Here's how the part is built. I have some questions about the finished solid (model axes, mm). A direction names the side the tool comes from. Round coordinates to 2 decimals unless told otherwise and drop trailing zeros. Write each loop counter-clockwise with the first axis right and the second up, starting at its lowest first coordinate (ties: lowest second). Pieces come first, ordered by that corner, then holes. Notation, with made-up numbers: (51.25, -36.75) -> (57.25, -36.75) arc R20 ccw to (57.25, -15.75) -> close; hole circle Ø10 at (82.5, -28.5). An arc over 180 degrees is marked (long way). Put each result on its own line as item: value. Start each with the question number.
1. I need wall thicknesses on probe 1 along X at (y, z) = (-22, 2.75); probe 2 along X at (y, z) = (-25, 3); probe 3 along X at (y, z) = (-21, 5.75). Which ranges of each line are inside material? Lowest first, please. Write a range as from..to.
2. For pin 1 (3 mm diameter, centred on x = -22.5, z = 5.5, fed in from -Y); pin 2 (1 mm diameter, centred on y = 20.5, z = 1, fed in from -X), each with a flat end and sliding along its axis, tell me the tip position at first contact or that it passes through.
3. Suppose I cut it at D-D (y = -5). Please give me the cut outline in (x, z).
4. Suppose I cut it at C-C (x = -43). Please give me the cut outline in (y, z).
5. Suppose I cut it at A-A (y = -29). Please give me the cut outline in (x, z), then the cut area to 3 significant figures.
6. Suppose I cut it at B-B (z = 2.75). Count the separate pieces of the cut face and the enclosed holes in it, then the cut area to 3 significant figures.
7. Which directions (+Z, -Z, +X, -X, +Y, -Y) give clear straight access to the entire face, cutting with the end or side of a thin tool? Please do faces 1 (the face through (10.76, 28.77, 3.45)), 2 (the face through (-10.886, 29.184, 3.451)), 3 (the face through (19.534, -23.699, 3.451)).
```python
from build123d import *

# Parameters (mm, degrees)
F0_R     = 11
F0_R_2   = 1.5
F1_DEPTH = 7


with BuildPart() as f1:
    # F0 (on Top) → F1 (new body)
    with BuildSketch(Plane.XY):
        with BuildLine():
            Line((-16.379662, 43.88667), (-5.236542, 14.062915))
            ThreePointArc((-5.236542, 14.062915), (-9.677134, 11.46123), (-12.976923, 7.51167))
            ThreePointArc((-12.976923, 7.51167), (-14.764123, 2.679089), (-14.810571, -2.473169))
            Line((-14.810571, -2.473169), (-46.21026, -7.734822))
            ThreePointArc((-46.21026, -7.734822), (-58.47355, -33.74418), (-29.81714, -36.128538))
            Line((-29.81714, -36.128538), (-9.560571, -11.566436))
            ThreePointArc((-9.560571, -11.566436), (-5.07992, -14.127023), (0.003377, -15.01749))
            ThreePointArc((0.003377, -15.01749), (5.073691, -14.134569), (9.547113, -11.589746))
            Line((9.547113, -11.589746), (29.803682, -36.151848))
            ThreePointArc((29.803682, -36.151848), (58.460092, -33.76749), (46.196802, -7.758132))
            Line((46.196802, -7.758132), (14.797113, -2.496479))
            ThreePointArc((14.797113, -2.496479), (14.77432, 2.664172), (13.003839, 7.51167))
            ThreePointArc((13.003839, 7.51167), (9.70405, 11.46123), (5.263458, 14.062915))
            Line((5.263458, 14.062915), (16.406578, 43.88667))
            ThreePointArc((16.406578, 43.88667), (0.013458, 67.51167), (-16.379662, 43.88667))
        make_face()
        with Locations((-43.318105, -24.99418)):
            Circle(F0_R, mode=Mode.SUBTRACT)
        with Locations((-25.49547, -22.305525)):
            Circle(F0_R_2, mode=Mode.SUBTRACT)
        with Locations((-32.045816, -10.959994)):
            Circle(F0_R_2, mode=Mode.SUBTRACT)
        with Locations((-17.676041, -10.205267)):
            Circle(F0_R_2, mode=Mode.SUBTRACT)
        with Locations((25.514541, -22.272493)):
            Circle(F0_R_2, mode=Mode.SUBTRACT)
        with Locations((43.304647, -25.01749)):
            Circle(F0_R, mode=Mode.SUBTRACT)
        with Locations((17.676041, -10.205267)):
            Circle(F0_R_2, mode=Mode.SUBTRACT)
        with Locations((0.013458, 0.01167)):
            Circle(F0_R, mode=Mode.SUBTRACT)
        with Locations((32.064887, -10.926962)):
            Circle(F0_R_2, mode=Mode.SUBTRACT)
        with Locations((-6.569416, 33.232488)):
            Circle(F0_R_2, mode=Mode.SUBTRACT)
        with Locations((0, 20.410534)):
            Circle(F0_R_2, mode=Mode.SUBTRACT)
        with Locations((6.531274, 33.232488)):
            Circle(F0_R_2, mode=Mode.SUBTRACT)
        with Locations((0.013458, 50.01167)):
            Circle(F0_R, mode=Mode.SUBTRACT)
    extrude(amount=F1_DEPTH)


solid = f1.part
```
Verdict:
1. probe 1: x = -60.56..-53.9, -32.73..-26.96, -24.03..-18.17, 18.13..24.04, 26.99..32.73, 53.88..60.54
1. probe 2: x = -60.82..-54.32, -32.32..-20.64, 20.61..32.3, 54.3..60.8
1. probe 3: x = -60.36..-53.57, -33.07..-26.23, -24.76..-17.34, 17.31..24.72, 26.31..33.06, 53.54..60.34
2. pin 1: stops at y = -29.07
2. pin 2: stops at x = -7.83
3. outline: (-29.89, 0) -> (-9.78, 0) -> (-9.78, 7) -> (-29.89, 7) -> close; (9.81, 0) -> (29.74, 0) -> (29.74, 7) -> (9.81, 7) -> close
4. outline: (-42.49, 0) -> (-35.99, 0) -> (-35.99, 7) -> (-42.49, 7) -> close; (-14, 0) -> (-7.2, 0) -> (-7.2, 7) -> (-14, 7) -> close
5. outline: (-60.35, 0) -> (-53.56, 0) -> (-53.56, 7) -> (-60.35, 7) -> close; (-33.07, 0) -> (-23.94, 0) -> (-23.94, 7) -> (-33.07, 7) -> close; (23.91, 0) -> (33.05, 0) -> (33.05, 7) -> (23.91, 7) -> close; (53.56, 0) -> (60.35, 0) -> (60.35, 7) -> (53.56, 7) -> close
5. area: 223 mm^2
6. separate pieces: 1
6. enclosed holes: 13
6. area: 3,110 mm^2
7. face 1: +Z, -Z, +X
7. face 2: +Z, -Z, -X
7. face 3: +Z, -Z, -Y
